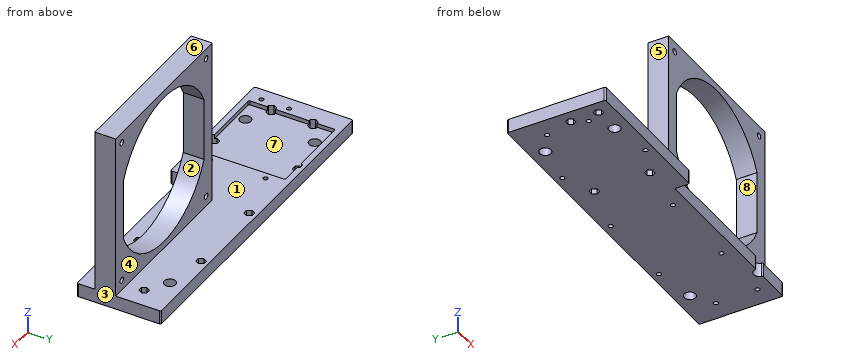
```python
from build123d import *

# Parameters (mm, degrees)
SKETCH1_R           = 4.1
SKETCH1_R_2         = 1.65
BOSS_EXTRUDE1_DEPTH = 10
CUT_EXTRUDE1_DEPTH  = 7
CUT_EXTRUDE2_DEPTH  = 3
CUT_EXTRUDE3_DEPTH  = 5
SKETCH5_W           = 120
SKETCH5_H           = 15
BOSS_EXTRUDE2_DEPTH = 120
SKETCH6_R           = 2.1
CUT_EXTRUDE4_DEPTH  = 15


with BuildPart() as part:
    # Sketch1 → Boss-Extrude1 (new body)
    with BuildSketch(Plane.XY):
        with BuildLine():
            Line((118.5, -25), (95.0009999, -25))
            ThreePointArc((95.0009999, -25), (94.366996127, -24.773329953), (94.020411684, -24.196078431))
            ThreePointArc((94.020411684, -24.196078431), (90, -20.9), (85.979588316, -24.196078431))
            ThreePointArc((85.979588316, -24.196078431), (85.633003873, -24.773329953), (84.9990001, -25))
            Line((84.9990001, -25), (-14, -25))
            ThreePointArc((-14, -25), (-14.707106781, -25.292893219), (-15, -26))
            Line((-15, -26), (-15, -34.5))
            ThreePointArc((-15, -34.5), (-15.292893219, -35.207106781), (-16, -35.5))
            Line((-16, -35.5), (-118.5, -35.5))
            ThreePointArc((-118.5, -35.5), (-119.207106781, -35.207106781), (-119.5, -34.5))
            Line((-119.5, -34.5), (-119.5, 34.5))
            ThreePointArc((-119.5, 34.5), (-119.207106781, 35.207106781), (-118.5, 35.5))
            Line((-118.5, 35.5), (118.5, 35.5))
            ThreePointArc((118.5, 35.5), (119.207106781, 35.207106781), (119.5, 34.5))
            Line((119.5, 34.5), (119.5, -24))
            ThreePointArc((119.5, -24), (119.207106781, -24.707106781), (118.5, -25))
        make_face()
        with Locations((-90, 25)):
            Circle(SKETCH1_R, mode=Mode.SUBTRACT)
        with Locations((90, 25)):
            Circle(SKETCH1_R, mode=Mode.SUBTRACT)
        with Locations((-90, -25)):
            Circle(SKETCH1_R, mode=Mode.SUBTRACT)
        with Locations((105, -15)):
            Circle(SKETCH1_R_2, mode=Mode.SUBTRACT)
        with Locations((-60, 30)):
            Circle(SKETCH1_R_2, mode=Mode.SUBTRACT)
        with Locations((-60, -30)):
            Circle(SKETCH1_R_2, mode=Mode.SUBTRACT)
        with Locations((-105, 15)):
            Circle(SKETCH1_R_2, mode=Mode.SUBTRACT)
        with Locations((-105, -15)):
            Circle(SKETCH1_R_2, mode=Mode.SUBTRACT)
        with Locations(Location((-37.5, 20, 0), (0, 0, 180))):
            Circle(SKETCH1_R_2, mode=Mode.SUBTRACT)
        with Locations(Location((-37.5, -20, 0), (0, 0, 180))):
            Circle(SKETCH1_R_2, mode=Mode.SUBTRACT)
        with Locations(Location((-110, -5.001676566, 0), (0, 0, 180))):
            Circle(SKETCH1_R_2, mode=Mode.SUBTRACT)
        with Locations(Location((-110, -25, 0), (0, 0, 180))):
            Circle(SKETCH1_R_2, mode=Mode.SUBTRACT)
        with Locations((60, 30)):
            Circle(SKETCH1_R_2, mode=Mode.SUBTRACT)
        with Locations((60, -15)):
            Circle(SKETCH1_R_2, mode=Mode.SUBTRACT)
        with Locations((105, 15)):
            Circle(SKETCH1_R_2, mode=Mode.SUBTRACT)
        with Locations((0, 30)):
            Circle(SKETCH1_R_2, mode=Mode.SUBTRACT)
        with Locations((0, -15)):
            Circle(SKETCH1_R_2, mode=Mode.SUBTRACT)
    extrude(amount=BOSS_EXTRUDE1_DEPTH)

    # Sketch2 → Cut-Extrude1 (cut)
    with BuildSketch(Plane.XY.offset(10)):
        Polygon((-101.651368439, 15), (-103.325684219, 17.9), (-106.674315781, 17.9), (-108.348631561, 15), (-106.674315781, 12.1), (-103.325684219, 12.1), align=None)
        Polygon((-101.651368439, -15), (-103.325684219, -12.1), (-106.674315781, -12.1), (-108.348631561, -15), (-106.674315781, -17.9), (-103.325684219, -17.9), align=None)
        Polygon((-56.651368439, 30), (-58.325684219, 32.9), (-61.674315781, 32.9), (-63.348631561, 30), (-61.674315781, 27.1), (-58.325684219, 27.1), align=None)
        Polygon((108.348631561, -15), (106.674315781, -12.1), (103.325684219, -12.1), (101.651368439, -15), (103.325684219, -17.9), (106.674315781, -17.9), align=None)
        Polygon((63.348631561, 30), (61.674315781, 32.9), (58.325684219, 32.9), (56.651368439, 30), (58.325684219, 27.1), (61.674315781, 27.1), align=None)
        Polygon((-56.651368439, -30), (-58.325684219, -27.1), (-61.674315781, -27.1), (-63.348631561, -30), (-61.674315781, -32.9), (-58.325684219, -32.9), align=None)
        Polygon((63.348631561, -15), (61.674315781, -12.1), (58.325684219, -12.1), (56.651368439, -15), (58.325684219, -17.9), (61.674315781, -17.9), align=None)
        Polygon((108.348631561, 15), (106.674315781, 17.9), (103.325684219, 17.9), (101.651368439, 15), (103.325684219, 12.1), (106.674315781, 12.1), align=None)
        Polygon((3.348631561, 30), (1.674315781, 32.9), (-1.674315781, 32.9), (-3.348631561, 30), (-1.674315781, 27.1), (1.674315781, 27.1), align=None)
        Polygon((3.348631561, -15), (1.674315781, -12.1), (-1.674315781, -12.1), (-3.348631561, -15), (-1.674315781, -17.9), (1.674315781, -17.9), align=None)
    extrude(amount=-CUT_EXTRUDE1_DEPTH, mode=Mode.SUBTRACT)

    # Sketch3 → Cut-Extrude2 (cut)
    with BuildSketch(Plane.XY.offset(10)):
        with BuildLine():
            Line((-104, 31.25), (-43.5, 31.25))
            ThreePointArc((-43.5, 31.25), (-42.792893219, 30.957106781), (-42.5, 30.25))
            Line((-42.5, 30.25), (-42.5, -30.25))
            ThreePointArc((-42.5, -30.25), (-42.792893219, -30.957106781), (-43.5, -31.25))
            Line((-43.5, -31.25), (-104, -31.25))
            ThreePointArc((-104, -31.25), (-104.707106781, -30.957106781), (-105, -30.25))
            Line((-105, -30.25), (-105, 30.25))
            ThreePointArc((-105, 30.25), (-104.707106781, 30.957106781), (-104, 31.25))
        make_face()
    extrude(amount=-CUT_EXTRUDE2_DEPTH, mode=Mode.SUBTRACT)

    # Sketch4 → Cut-Extrude3 (cut)
    with BuildSketch(Plane(origin=(0, 0, 0), x_dir=(-1, 0, 0), z_dir=(0, 0, -1))):
        Polygon((40.848631561, 20), (39.174315781, 22.9), (35.825684219, 22.9), (34.151368439, 20), (35.825684219, 17.1), (39.174315781, 17.1), align=None)
        Polygon((40.848631561, -20), (39.174315781, -17.1), (35.825684219, -17.1), (34.151368439, -20), (35.825684219, -22.9), (39.174315781, -22.9), align=None)
        Polygon((113.348631561, -25), (111.674315781, -22.1), (108.325684219, -22.1), (106.651368439, -25), (108.325684219, -27.9), (111.674315781, -27.9), align=None)
        Polygon((113.348631561, -5.001676566), (111.674315781, -2.101676566), (108.325684219, -2.101676566), (106.651368439, -5.001676566), (108.325684219, -7.901676566), (111.674315781, -7.901676566), align=None)
    extrude(amount=-CUT_EXTRUDE3_DEPTH, mode=Mode.SUBTRACT)

    # Sketch5 → Boss-Extrude2 (add)
    with BuildSketch(Plane.XY.offset(10)):
        with Locations((59.5, -4.6)):
            Rectangle(SKETCH5_W, SKETCH5_H)
    extrude(amount=BOSS_EXTRUDE2_DEPTH)

    # Sketch6 → Cut-Extrude4 (cut)
    with BuildSketch(Plane.XZ.offset(12.1)):
        with Locations(Location((7, 122.5, 0), (0, 0, 270))):
            Circle(SKETCH6_R)
        with Locations(Location((7, 17.5, 0), (0, 0, 270))):
            Circle(SKETCH6_R)
        with Locations(Location((112, 17.5, 0), (0, 0, 270))):
            Circle(SKETCH6_R)
        with Locations(Location((112, 122.5, 0), (0, 0, 270))):
            Circle(SKETCH6_R)
        with BuildLine():
            Line((9.5, 92.912878475), (9.5, 47.087121525))
            ThreePointArc((9.5, 47.087121525), (59.5, 15), (109.5, 47.087121525))
            Line((109.5, 47.087121525), (109.5, 92.912878475))
            ThreePointArc((109.5, 92.912878475), (59.5, 125), (9.5, 92.912878475))
        make_face()
    extrude(amount=-CUT_EXTRUDE4_DEPTH, mode=Mode.SUBTRACT)


solid = part.part
```
The listing builds one solid part. Answer for the finished solid, in the listing's coordinates (mm). Face numbers are marked on the shaded views. A direction names the side the tool comes from. Round coordinates to 2 decimals unless told otherwise and drop trailing zeros. Write each loop counter-clockwise with the first axis right and the second up, starting at its lowest first coordinate (ties: lowest second). Pieces come first, ordered by that corner, then holes. Notation, with made-up numbers: (87, -27.75) -> (102, -27.75) arc R11 cw to (102, -9.75) -> close; hole circle Ø10 at (70.5, -37). An arc over 180 degrees is marked (long way). Answer as a JSON object with one key per item and string values. Group by question number.
Q1. Section A-A (z = 88.5) is taken. Write down the section's boundary in (x, y).
Q2. Determine the mould class of the marked faces 1, 2 and 3 for opening direction X: pulls with the +X half, pulls with the -X half, needs draft (parallel to the pull), parting line crosses it, or undercut.
Q3. Straight lines are drawn through the part: line 1 along Y through (x, z) = (-105, 0.8); line 2 along X through (y, z) = (-20, 8.55); line 3 along Y through (x, z) = (60, 2.25). For each, find the intervals that lie inside material, in ascending order.
Q4. Section B-B (x = 26) is taken. Write down the section's boundary in (y, z), plus the area to 3 significant figures.
Q5. Which of the six approach directions +Z, -Z, +X, -X, +Y, -Y give full straight-line access (tool end or side, diameter ignored) to the marked faces 4, 5, 6, 7 and 8?
Q6. Section D-D (x = -71) is taken. Write down the section's boundary in (y, z).
Q7. Each of these flat-tipped pins is pushed along its axis until it touches: pin 1 Ø1.7 at (x, z) = (105, 5) entering from -Y; pin 2 Ø4 at (y, z) = (-29, 5.5) entering from +X; pin 3 Ø5 at (x, z) = (112, 17.5) entering from -Y. Where does it stop, or does it pass through?
Q8. Section C-C (y = 7.5) is taken. Write down the section's boundary in (x, z).
Check values:
{
 "1": {"outline": "(-0.5, -12.1) -> (9.5, -12.1) -> (9.5, 2.9) -> (-0.5, 2.9) -> close; (109.5, -12.1) -> (119.5, -12.1) -> (119.5, 2.9) -> (109.5, 2.9) -> close"},
 "2": {"face 1": "needs draft", "face 2": "undercut", "face 3": "pulls with the +X half"},
 "3": {"line 1": "-35.5 to -16.65, -13.35 to 13.35, 16.65 to 35.5", "line 2": "-119.5 to -105, -42.5 to -39.15, -35.85 to 119.5", "line 3": "-25 to -16.65, -13.35 to 28.35, 31.65 to 35.5"},
 "4": {"outline": "(-25, 0) -> (35.5, 0) -> (35.5, 10) -> (2.9, 10) -> (2.9, 26.38) -> (-12.1, 26.38) -> (-12.1, 10) -> (-25, 10) -> close; (-12.1, 113.62) -> (2.9, 113.62) -> (2.9, 130) -> (-12.1, 130) -> close", "area": "1,100 mm^2"},
 "5": {"face 4": "+Z, +X, -X, +Y", "face 5": "+Z, -X, +Y, -Y", "face 6": "+Z, +X, -X, +Y, -Y", "face 7": "+Z", "face 8": "+Y, -Y"},
 "6": {"outline": "(-35.5, 0) -> (35.5, 0) -> (35.5, 10) -> (31.25, 10) -> (31.25, 7) -> (-31.25, 7) -> (-31.25, 10) -> (-35.5, 10) -> close"},
 "7": {"pin 1": "y = -25", "pin 2": "x = -15", "pin 3": "y = -12.1"},
 "8": {"outline": "(-119.5, 0) -> (119.5, 0) -> (119.5, 10) -> (-42.5, 10) -> (-42.5, 7) -> (-105, 7) -> (-105, 10) -> (-119.5, 10) -> close"}
}
